Part model, mm, in its own coordinate system. Face numbers are marked on the shaded views. A direction names the side the tool comes from. Round coordinates to 2 decimals unless told otherwise and drop trailing zeros. Loops run counter-clockwise (first coordinate to the right, second up) from the corner with the lowest first, then second, coordinate; pieces in that order, holes last. Notation, with made-up numbers: (-19, 83.25) -> (-2, 83.25) arc R27 ccw to (-2, 100.25) -> close; hole circle Ø1 at (38, -26.5). An arc over 180 degrees is marked (long way). Use a Markdown table: item, result. Add a question column.
Item 1: Two-plate mould, pull along Y, no slides. Class the marked faces 6, 7 and 8: pulls with the +Y half, pulls with the -Y half, needs draft (parallel to the pull), parting line crosses it, or undercut.
Item 2: Flat gauge pins, fed straight in: pin 1 (7.5 mm diameter, centred on x = 0.5, y = -70, fed in from +Z); pin 2 (20.5 mm diameter, centred on y = -40, z = 15, fed in from +X); pin 3 (12 mm diameter, centred on x = -41.74, y = -21.94, fed in from +Z); pin 4 (7.5 mm diameter, centred on y = -56.5, z = 6.5, fed in from -X). Where does each tip first touch, or does it go through?
Item 3: Cut at B-B, the plane y = -92.5. List the corners of the cut face in (x, z), plus the area to 3 significant figures.
Item 4: Cut at C-C, the plane x = -36.5. List the corners of the cut face in (y, z), plus the area to 3 significant figures.
Item 5: Cut at D-D, the plane x = -81.5. List the corners of the cut face in (y, z).
Item 6: Probe line 1 (Y direction, x = -44, z = 12); line 2 (X direction, y = -37, z = -24.5); line 3 (Z direction, x = -48.5, y = -40). List the from-to ranges inside material, lowest first. Write a range as [from, to].
Item 7: Cut at A-A, the plane z = -24. List the corners of the cut face in (x, y), plus the area to 3 significant figures.
Item 8: Which spindle directions (+Z, -Z, +X, -X, +Y, -Y) get a long thin tool onto all of the face, cutting with end or side? Do the marked faces 1, 2, 3, 4 and 5. Say none if no direction does.
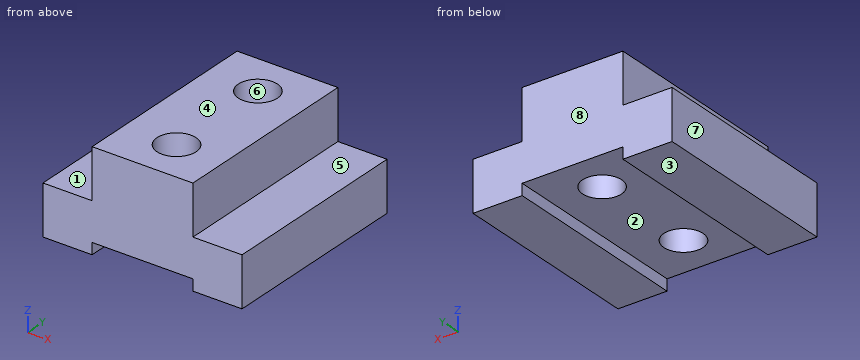
```python
from build123d import *

# Parameters (mm, degrees)
F1_DEPTH = 100
F3_D     = 20


with BuildPart() as f1:
    # F0 (on Front) → F1 (new body)
    with BuildSketch(Plane.XZ):
        Polygon((-17.148554, -2.782671), (-17.148554, 22.617329), (-42.870075, 22.617329), (-42.870075, -22.395332), (-17.148554, -22.395332), (-17.148554, -28.182671), (7.929928, -28.182671), (7.929928, -2.782671), align=None)
        Polygon((-42.870075, -22.395332), (-42.870075, 22.617329), (-68.591596, 22.617329), (-68.591596, -2.782671), (-93.670078, -2.782671), (-93.670078, -28.182671), (-68.591596, -28.182671), (-68.591596, -22.395332), align=None)
    extrude(amount=F1_DEPTH)

    # F3 (through all)
    with Locations(Plane.XY.offset(22.617329)):
        with Locations((-41.735466, -21.940365), (-41.735466, -78.059635)):
            Hole(F3_D / 2)


solid = f1.part
```
A:
| question | item | result |
|---|---|---|
| 1 | face 6 | undercut |
| 1 | face 7 | needs draft |
| 1 | face 8 | pulls with the +Y half |
| 2 | pin 1 | stops at z = -2.78 |
| 2 | pin 2 | stops at x = -17.15 |
| 2 | pin 3 | passes through |
| 2 | pin 4 | stops at x = -68.59 |
| 3 | outline | (-93.67, -28.18) -> (-68.59, -28.18) -> (-68.59, -22.4) -> (-17.15, -22.4) -> (-17.15, -28.18) -> (7.93, -28.18) -> (7.93, -2.78) -> (-17.15, -2.78) -> (-17.15, 22.62) -> (-68.59, 22.62) -> (-68.59, -2.78) -> (-93.67, -2.78) -> close |
| 3 | area | 3,590 mm^2 |
| 4 | outline | (-100, -22.4) -> (-86.58, -22.4) -> (-86.58, 22.62) -> (-100, 22.62) -> close; (-69.54, -22.4) -> (-30.46, -22.4) -> (-30.46, 22.62) -> (-69.54, 22.62) -> close; (-13.42, -22.4) -> (0, -22.4) -> (0, 22.62) -> (-13.42, 22.62) -> close |
| 4 | area | 2,970 mm^2 |
| 5 | outline | (-100, -28.18) -> (0, -28.18) -> (0, -2.78) -> (-100, -2.78) -> close |
| 6 | line 1 | y = [-100, -87.8], [-68.32, -31.68], [-12.2, 0] |
| 6 | line 2 | x = [-93.67, -68.59], [-17.15, 7.93] |
| 6 | line 3 | z = [-22.4, 22.62] |
| 7 | outline | (-93.67, -100) -> (-68.59, -100) -> (-68.59, 0) -> (-93.67, 0) -> close; (-17.15, -100) -> (7.93, -100) -> (7.93, 0) -> (-17.15, 0) -> close |
| 7 | area | 5,020 mm^2 |
| 8 | face 1 | +Z, -X, +Y, -Y |
| 8 | face 2 | -Z, +Y, -Y |
| 8 | face 3 | -Z, +X, -X, +Y, -Y |
| 8 | face 4 | +Z, +X, -X, +Y, -Y |
| 8 | face 5 | +Z, +X, +Y, -Y |
